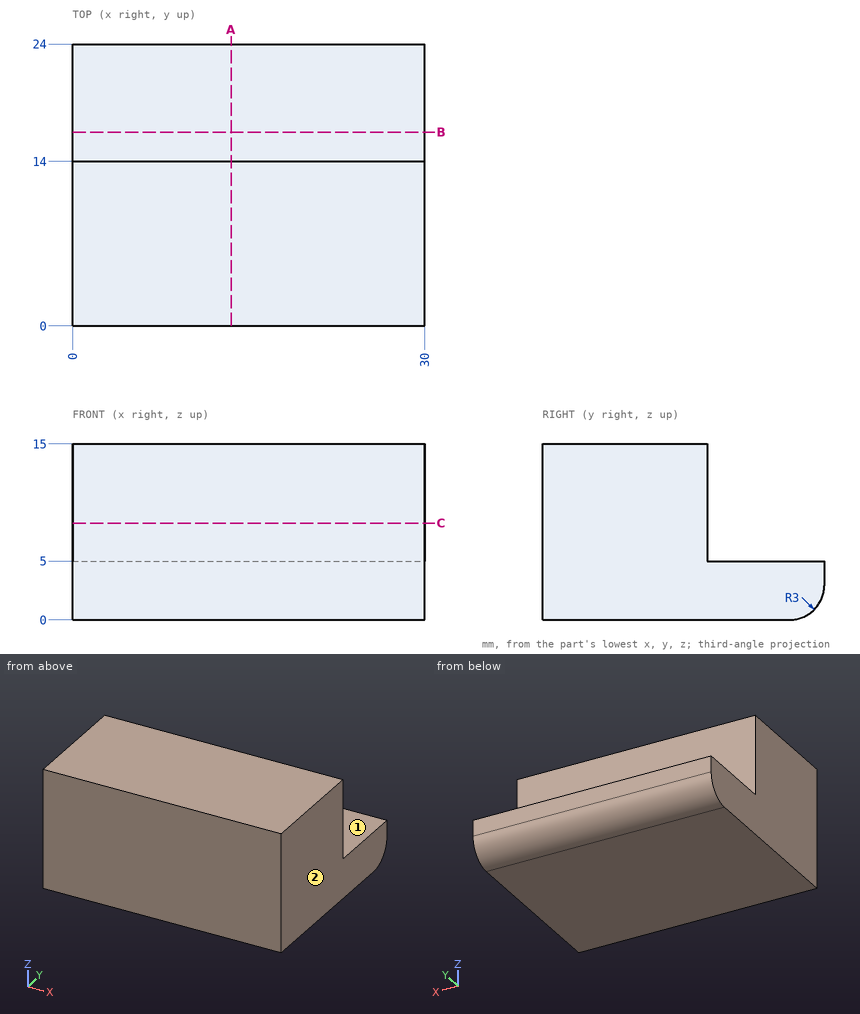
Part print with two shaded views. Sizes in mm from the minimum x, y, z corner. A direction names the side the tool comes from. Coordinates: 2 decimals unless noted, no trailing zeros. Order: outer loops, then holes, each group sorted by start corner. A loop starts at its lowest first (then second) coordinate and runs counter-clockwise, first axis right, second up. Notation, with made-up numbers: M -22.5,15 L -16.5,15 A13 cw -16.5,36 Z; hole C 10,79.25 d11. An arc over 180 degrees is marked long. One line per question, with ' | ' between items. Start each with the question number.
1. Cut at A-A (x = 13.5). Write the cut outline in (y, z).
2. Wall check: line 1 along Y through (x, z) = (7.5, 10); line 2 along Z through (x, y) = (11, 18.5); line 3 along Z through (x, y) = (3.5, 23.25). Give the ranges that are in metal, low to high. Write a range as [from, to].
3. Cut at B-B (y = 16.5). Write the cut outline in (x, z).
4. Tool access for the marked faces 1 and 2: list every direction of +Z, -Z, +X, -X, +Y, -Y with a clear straight run to the whole face (end or side of a thin tool).
5. Flat gauge pins, fed straight in: P1, Ø8, axis at x = 17.5, z = 11.5, coming from the +Y side; P2, Ø4, axis at x = 7.5, y = 19.5, coming from the +Z side. Where does each tip first touch, or does it go through?
6. Cut at C-C (z = 8.25). Write the cut outline in (x, y).
The answers:
1) outline: M 0,0 L 21,0 A3 ccw 24,3 L 24,5 L 14,5 L 14,15 L 0,15 Z
2) line 1: y = [0, 14] | line 2: z = [0, 5] | line 3: z = [1.02, 5]
3) outline: M 0,0 L 30,0 L 30,5 L 0,5 Z
4) face 1: +Z, +X, -X, +Y | face 2: +Z, -Z, +X, +Y, -Y
5) P1: stops at y = 14 | P2: stops at z = 5
6) outline: M 0,0 L 30,0 L 30,14 L 0,14 Z
